from build123d import *

# Parameters (mm, degrees)
CUT_EXTRUDE1_DEPTH = 4


with BuildPart() as part:
    # Sketch1 → Revolve1 (revolve)
    with BuildSketch(Plane(origin=(0, 0, 0), x_dir=(0, 0, -1), z_dir=(1, 0, 0))):
        Polygon((-5, 0), (-5, 3), (81.2, 3), (81.2, 8), (85.2, 8), (85.2, 0), align=None)
    revolve(axis=Axis((0, 0, -85.2), (0, 0, 1)))

    # Sketch2 → Revolve2 (revolve)
    with BuildSketch(Plane(origin=(0, 0, 0), x_dir=(0, 0, -1), z_dir=(1, 0, 0))):
        with BuildLine():
            Line((-21, 0), (-21, 2.3865))
            Line((-21, 2.3865), (-20.3865, 3))
            Line((-20.3865, 3), (-8.148486452, 3))
            Line((-8.148486452, 3), (-6.599415898, 2.436184428))
            ThreePointArc((-6.599415898, 2.436184428), (-6.498392718, 2.409115348), (-6.394203812, 2.4))
            Line((-6.394203812, 2.4), (-5.6, 2.4))
            ThreePointArc((-5.6, 2.4), (-5.175735931, 2.575735931), (-5, 3))
            Line((-5, 3), (-4, 3))
            Line((-4, 3), (-4, 0))
            Line((-4, 0), (-21, 0))
        make_face()
    revolve(axis=Axis((0, 0, 4), (0, 0, 1)))

    # Sketch3 → Cut-Extrude1 (cut)
    with BuildSketch(Plane.XY.offset(2)):
        Polygon((-5, 10), (-5, -5), (-2.5, -5), (-2.5, 5), (2.5, 5), (2.5, -5), (5, -5), (5, 10), align=None)
    extrude(amount=CUT_EXTRUDE1_DEPTH, mode=Mode.SUBTRACT)


solid = part.part
Can you work these out from the model? Positions are in its coordinate system, mm. A direction names the side the tool comes from. Give positions to 0.01 mm unless a question says otherwise; leave off trailing zeros. Order: outer loops, then holes, each group sorted by start corner. A loop starts at its lowest first (then second) coordinate and runs counter-clockwise, first axis right, second up. Notation, with made-up numbers: M 49.5,76.5 L 96.5,76.5 A7 ccw 96.5,83.5 Z; hole C 67.5,50.5 d1. An arc over 180 degrees is marked long. One line per question, with ' | ' between items.
Item 1: We'd pull the mould along Z, two halves only. Please class faces 1 (the face through (7.81, -1.73, -83.23)), 2 (the face through (0, 0, -85.2)), 3 (the face through (-2.5, 0, 4)), 4 (the face through (-0.1, -3.4, -81.2)): released by +Z, released by -Z, zero draft, split by the parting line, or undercut.
Answer block:
face 1: zero draft | face 2: released by -Z | face 3: undercut | face 4: released by +Z
Item 2: Suppose I cut it at B-B, the plane x = 0. Write out the boundary of the cut face in (y, z).
Answer block:
outline: M -8,-85.2 L 8,-85.2 L 8,-81.2 L 3,-81.2 L 3,5 A0.6 cw 2.4,5.6 L 2.4,6.39 A0.6 cw 2.44,6.6 L 3,8.15 L 3,20.39 L 2.39,21 L -2.39,21 L -3,20.39 L -3,8.15 L -2.44,6.6 A0.6 cw -2.4,6.39 L -2.4,5.6 A0.6 cw -3,5 L -3,-81.2 L -8,-81.2 Z
Item 3: Suppose I cut it at C-C, the plane z = -28.5. Write out the boundary of the cut face in (x, y).
Answer block:
outline: C 0,0 d6
Item 4: Please list where these lines run through material, in increasing order: L1, parallel to Z at x = -6.5, y = -4.25; L2, parallel to Z at x = 2.25, y = -1.5; L3, parallel to X at y = -0.75, z = -34.
Answer block:
L1: z = -85.2 to -81.2 | L2: z = -85.2 to 5.08, 7.34 to 20.68 | L3: x = -2.9 to 2.9
Item 5: Suppose I cut it at A-A, the plane y = 0. Write out the boundary of the cut face in (x, z).
Answer block:
outline: M -8,-85.2 L 8,-85.2 L 8,-81.2 L 3,-81.2 L 3,2 L 2.5,2 L 2.5,5.27 A0.6 cw 2.4,5.6 L 2.4,6.39 A0.6 cw 2.44,6.6 L 3,8.15 L 3,20.39 L 2.39,21 L -2.39,21 L -3,20.39 L -3,8.15 L -2.44,6.6 A0.6 cw -2.4,6.39 L -2.4,5.6 A0.6 cw -2.5,5.27 L -2.5,2 L -3,2 L -3,-81.2 L -8,-81.2 Z
Item 6: Suppose I cut it at D-D, the plane y = 4. Write out the boundary of the cut face in (x, z), then the cut area to 3 significant figures.
Answer block:
outline: M -6.93,-85.2 L 6.93,-85.2 L 6.93,-81.2 L -6.93,-81.2 Z | area: 55.4 mm2
Item 7: For faces 5 (the face through (2.5, 0, 4)), 6 (the face through (0, -3, -39)), 7 (the face through (-2.024, 1.29, 5.992)), which set-ups out of +Z, -Z, +X, -X, +Y, -Y let a thin tool reach every point of the face, with its end or its side?
Answer block:
face 5: +X, +Y, -Y | face 6: +Z | face 7: none
Item 8: I'm going to push flat-ended pins straight in: pin 1 Ø2 at (x, y) = (-4, 2) entering from +Z; pin 2 Ø4 at (y, z) = (-1, -61) entering from -X; pin 3 Ø1.5 at (x, z) = (-3, -68.5) entering from +Y. Where does each tip first touch, or does it pass through?
Answer block:
pin 1: stops at z = -81.2 | pin 2: stops at x = -3 | pin 3: stops at y = 1.98
